Autodesk Inventor part; units mm, degrees
ref_plane "YZ Plane" through (0, 0, 0) normal (1, 0, 0) x (0, 1, 0)
ref_plane "XZ Plane" through (0, 0, 0) normal (0, 1, 0) x (-1, 0, 0)
ref_plane "XY Plane" through (0, 0, 0) normal (0, 0, 1) x (1, 0, 0)
sketch "Sketch1" plane through (0, 0, 0) normal (0, 0, 1) x (1, 0, 0)
  circle A0 centre (0, 0) radius 5
  circle A1 centre (0, 0) radius 8
  line L0 (0, 13) -> (20, 13)
  line L1 (20, 13) -> (20, 2)
  line L2 (10, -8) -> (5, -13)
  line L3 (5, -13) -> (0, -13)
  line L4 (10, -8) -> (19, -8)
  line L5 (19, -8) -> (19, 1)
  line L6 (19, 1) -> (20, 2)
  line L7 (0, 19.5854) -> (0, -21.9543) construction
  line L8 (0, 13) -> (-20, 13)
  line L9 (-20, 13) -> (-20, 2)
  line L10 (-10, -8) -> (-5, -13)
  line L11 (-5, -13) -> (0, -13)
  line L12 (-10, -8) -> (-19, -8)
  line L13 (-19, -8) -> (-19, 1)
  line L14 (-19, 1) -> (-20, 2)
  dimension "d0" = 10
  dimension "d8" = 16
  dimension "d27" = 20
  dimension "d28" = 0
  dimension "d29" = 0
  dimension "d30" = 135
  dimension "d31" = 26
  dimension "d32" = 13
  dimension "d34" = 21
  dimension "d35" = 135
  dimension "d36" = 12
  dimension "d37" = 19
  dimension "d38" = 5
  dimension "d39" = 0
extrude "Extrusion1" add sketch "Sketch1" along normal blind 35 contours A1 | L0 L1 L6 L5 L4 L2 L3 L11 L10 L12 L13 L14 L9 L8
chamfer "Chamfer1" distance 1 angle 45 2 edges at (19, -8, 17.5) (-19, -8, 17.5)
sketch "Sketch3" plane through (-20, 13, 0) normal (0, 1, 0) x (1, 0, 0)
  line L0 (40, 0) -> (0, 0)
  line L1 (0, 0) -> (0, -35)
  line L2 (40, -35) -> (0, -35)
  line L3 (40, 0) -> (40, -35)
  point P0 (20, 0)
  point P1 (6, -27.5)
  point P2 (6, -7.5)
  point P3 (34, -27.5)
  point P4 (34, -7.5)
  dimension "d45" = 20
  dimension "d48" = 28
  dimension "d51" = 6
  dimension "d52" = 7.5
hole "Hole2" at (-14, 13, 27.5) at (-14, 13, 7.5) at (14, 13, 27.5) at (14, 13, 7.5) direction (0, -1, 0) diameter 3.242 end through all
properties part number "LinearBearing_SC10UU"
Can you work these out from the model? Positions are in its coordinate system, mm. A direction names the side the tool comes from. Coordinates: 2 decimals unless noted, no trailing zeros. Write each loop counter-clockwise with the first axis right and the second up, starting at its lowest first coordinate (ties: lowest second). Pieces come first, ordered by that corner, then holes. Notation, with made-up numbers: (53.5, 16) -> (64.5, 16) arc R17 ccw to (64.5, 24) -> close; hole circle Ø4 at (85.25, 20). An arc over 180 degrees is marked (long way). Write each question's results on one line, items separated by ' | '. Start each with the question number.
Q1. If I drill on probe 1 along X at (y, z) = (6, 27.5); probe 2 along Z at (x, y) = (-14, 7); probe 3 along X at (y, z) = (-0.25, 7.5), over which ranges is the centre line in solid material (lowest first)?
Q2. Imagine slicing it at D-D (x = -14). Write out the boundary of the cut face in (y, z), then the cut area to 3 significant figures.
Q3. Imagine slicing it at A-A (y = 0). Write out the boundary of the cut face in (x, z), then the cut area to 3 significant figures.
Q4. I'm going to push flat-ended pins straight in: pin 1 (1.5 mm diameter, centred on x = -8.5, z = 12, fed in from -Y); pin 2 (2.5 mm diameter, centred on x = -14, z = 7.5, fed in from -Y); pin 3 (2 mm diameter, centred on x = -14.5, z = 18, fed in from -Y); pin 4 (5 mm diameter, centred on y = -2, z = 15.5, fed in from +X). Where does each tip first touch, or does it pass through?
Q5. We'd pull the mould along X, two halves only. Please class faces 1 (the face through (13.93, 2.35, 25.88)), 2 (the face through (-1.08, 4.88, 17.26)), 3 (the face through (19, -3, 17)), 4 (the face through (0, 6, 35)): +X half, -X half, draft (parallel to the pull), parting line (faces both ways), or undercut.
Q6. On a 3-axis mill with a long thin cutter (end or side, diameter ignored), from which of +Z, -Z, +X, -X, +Y, -Y can I reach the whole of each face in a straight line? I mean faces 5 (the face through (-14.07, 2.35, 25.88)), 6 (the face through (-14, -8, 17)), 7 (the face through (14, -8, 17)). Say none if no direction works.
Q7. Imagine slicing it at C-C (z = 19.5). Write out the boundary of the cut face in (x, y).
Q8. Imagine slicing it at B-B (x = 0). Write out the boundary of the cut face in (y, z).
Taken from the geometry:
1) probe 1: x = -20 to -15.62, -12.38 to 12.38, 15.62 to 20 | probe 2: z = 0 to 5.88, 9.12 to 25.88, 29.12 to 35 | probe 3: x = -19 to -15.62, -12.38 to -4.99, 4.99 to 12.38, 15.62 to 19
2) outline: (-8, 0) -> (13, 0) -> (13, 5.88) -> (-8, 5.88) -> close; (-8, 9.12) -> (13, 9.12) -> (13, 25.88) -> (-8, 25.88) -> close; (-8, 29.12) -> (13, 29.12) -> (13, 35) -> (-8, 35) -> close | area: 599 mm^2
3) outline: (-19, 0) -> (-5, 0) -> (-5, 35) -> (-19, 35) -> close; (5, 0) -> (19, 0) -> (19, 35) -> (5, 35) -> close; hole circle Ø3.24 at (-14, 7.5); hole circle Ø3.24 at (-14, 27.5); hole circle Ø3.24 at (14, 7.5); hole circle Ø3.24 at (14, 27.5) | area: 947 mm^2
4) pin 1: stops at y = -10.25 | pin 2: passes through | pin 3: stops at y = -8 | pin 4: stops at x = 19
5) face 1: undercut | face 2: undercut | face 3: +X half | face 4: draft
6) face 5: +Y, -Y | face 6: +Z, -Z, -X, -Y | face 7: +Z, -Z, +X, -Y
7) outline: (-20, 2) -> (-19, 1) -> (-19, -7) -> (-18, -8) -> (-10, -8) -> (-5, -13) -> (5, -13) -> (10, -8) -> (18, -8) -> (19, -7) -> (19, 1) -> (20, 2) -> (20, 13) -> (-20, 13) -> close; hole circle Ø10 at (0, 0)
8) outline: (-13, 0) -> (-5, 0) -> (-5, 35) -> (-13, 35) -> close; (5, 0) -> (13, 0) -> (13, 35) -> (5, 35) -> close
